Check sheet for the modelled part. Datum: model origin and axes. Units: mm. A direction names the side the tool comes from. Round coordinates to 2 decimals unless told otherwise and drop trailing zeros. Order: outer loops, then holes, each group sorted by start corner. A loop starts at its lowest first (then second) coordinate and runs counter-clockwise, first axis right, second up.
```python
from build123d import *

# Parameters (mm, degrees)
F0_R     = 15
F0_W     = 32
F0_H     = 70
F1_DEPTH = 30
F2_W     = 64
F2_H     = 70
F3_DEPTH = 10
F4_W     = 64
F4_H     = 70
F5_DEPTH = 10


with BuildPart() as f1:
    # F0 (on Front) → F1 (new body)
    with BuildSketch(Plane.XZ):
        with BuildLine():
            Line((-32, -35), (-32, 35))
            Line((-32, 35), (-60, 35))
            ThreePointArc((-60, 35), (-84.7487373415, 24.7487373415), (-95, 0))
            ThreePointArc((-95, 0), (-84.7487373415, -24.7487373415), (-60, -35))
            Line((-60, -35), (-32, -35))
        make_face()
        with Locations((-60, 0)):
            Circle(F0_R, mode=Mode.SUBTRACT)
        with Locations((-16, 0)):
            Rectangle(F0_W, F0_H)
        with Locations((16, 0)):
            Rectangle(F0_W, F0_H)
        with BuildLine():
            ThreePointArc((95, 0), (84.7487373415, 24.7487373415), (60, 35))
            Line((60, 35), (32, 35))
            Line((32, 35), (32, -35))
            Line((32, -35), (60, -35))
            ThreePointArc((60, -35), (84.7487373415, -24.7487373415), (95, 0))
        make_face()
        with Locations((60, 0)):
            Circle(F0_R, mode=Mode.SUBTRACT)
    extrude(amount=F1_DEPTH)

    # F2 (on face) → F3 (cut)
    with BuildSketch(Plane.XZ.offset(30)):
        Rectangle(F2_W, F2_H)
    extrude(amount=-F3_DEPTH, mode=Mode.SUBTRACT)

    # F4 (on face) → F5 (join)
    with BuildSketch(Plane(origin=(0, 0, 0), x_dir=(-1, 0, 0), z_dir=(0, 1, 0))):
        Rectangle(F4_W, F4_H)
    extrude(amount=F5_DEPTH)


solid = f1.part
```
Item 1: Sectioned sample at B-B (z = 11). Record the cut outline in (x, y).
Answer:
outline: (-93.23, -30) - (-70.2, -30) - (-70.2, 0) - (-93.23, 0) - close; (-49.8, -30) - (-32, -30) - (-32, -20) - (32, -20) - (32, -30) - (49.8, -30) - (49.8, 0) - (32, 0) - (32, 10) - (-32, 10) - (-32, 0) - (-49.8, 0) - close; (70.2, -30) - (93.23, -30) - (93.23, 0) - (70.2, 0) - close
Item 2: Sectioned sample at C-C (x = -67). Record the cut outline in (y, z).
Answer:
outline: (-30, -34.29) - (0, -34.29) - (0, -13.27) - (-30, -13.27) - close; (-30, 13.27) - (0, 13.27) - (0, 34.29) - (-30, 34.29) - close
Item 3: Sectioned sample at D-D (z = 28). Record the cut outline in (x, y).
Answer:
outline: (-81, -30) - (-32, -30) - (-32, -20) - (32, -20) - (32, -30) - (81, -30) - (81, 0) - (32, 0) - (32, 10) - (-32, 10) - (-32, 0) - (-81, 0) - close
Item 4: Access from +Z, -Z, +X, -X, +Y, -Y to the whole of each face (thin tool, end or side, straight path). Record for faces 1 (the flat face through (63, -30, 16)), 2 (the flat face through (32, -25, 0)), 3 (the flat face through (-32, 5, 0)), 4 (the flat face through (63, 0, 16)).
Answer:
face 1: +Z, -Z, +X, -X, -Y
face 2: +Z, -Z, -Y
face 3: +Z, -Z, -X, +Y
face 4: +Z, -Z, +X, +Y
Item 5: Sectioned sample at A-A (y = -4). Record the cut outline in (x, z), and give its area (3 significant figures).
Answer:
outline: (-60, -35) - (60, -35) arc R35 ccw to (60, 35) - (-60, 35) arc R35 ccw to start; hole circle Ø30 at (-60, 0); hole circle Ø30 at (60, 0)
area: 10,800 mm2
Item 6: Release check for a two-part mould opening along X. For faces 5 (the flat face through (-64, 0, 16)), 6 (the flat face through (32, 5, 0)), 7 (the cylindrical face through (45.015, -14.79, 0.66)) record: released by +X, released by -X, zero draft, split by the parting line, or undercut.
Answer:
face 5: zero draft
face 6: released by +X
face 7: undercut
Item 7: Go/stop test with flat-tipped pins: P1, Ø1, axis at y = -9, z = 19, coming from the +X side; P2, Ø1, axis at y = -21.5, z = 26.5, coming from the -X side; P3, Ø8, axis at x = 8, z = -20, coming from the -Y side; P4, Ø3, axis at y = -25, z = -1, coming from the +X side. Record where each tip stops, or that it passes through.
Answer:
P1: stops at x = 89.71
P2: stops at x = -83.43
P3: stops at y = -20
P4: stops at x = 95
Item 8: Scan lines: line 1 along Z through (x, y) = (-60, -20.5); line 2 along X through (y, z) = (-1, 1); line 3 along X through (y, z) = (-15.5, -4). Record each from-to range of solid material in increasing order.
Answer:
line 1: z = -35 to -15, 15 to 35
line 2: x = -94.99 to -74.97, -45.03 to 45.03, 74.97 to 94.99
line 3: x = -94.77 to -74.46, -45.54 to 45.54, 74.46 to 94.77
